from build123d import *

# Parameters (mm, degrees)
SKETCH1_R                = 13.8176
SKETCH1_R_2              = 12.7
BOSS_EXTRUDE1_DEPTH      = 16.5
SKETCH2_R                = 13.8176
BOSS_EXTRUDE2_DEPTH      = 4.318
CUT_EXTRUDE1_DEPTH       = 4.318
CIRPATTERN1_COUNT        = 6
CHAMFER1_SIZE            = 1.524
SKETCH4_R                = 4.5
BOSS_EXTRUDE3_DEPTH      = 1.5
SKETCH5_R                = 1.5875
BOSS_EXTRUDE4_DEPTH      = 0.5
BOSS_EXTRUDE4_DEPTH_BACK = 26


with BuildPart() as part:
    # Sketch1 → Boss-Extrude1 (new body)
    with BuildSketch(Plane(origin=(0, 0, 0), x_dir=(1, 0, 0), z_dir=(0, 1, 0))):
        with Locations(Location((0, 0, 0), (0, 0, 270))):  # turned: the seam where the file's is
            Circle(SKETCH1_R)
        with Locations(Location((0, 0, 0), (0, 0, 270))):  # turned: the seam where the file's is
            Circle(SKETCH1_R_2, mode=Mode.SUBTRACT)
    extrude(amount=BOSS_EXTRUDE1_DEPTH)

    # Sketch2 → Boss-Extrude2 (add)
    with BuildSketch(Plane(origin=(0, 16.5, 0), x_dir=(-1, 0, 0), z_dir=(0, 1, 0))):
        with Locations(Location((0, 0, 0), (0, 0, 90))):  # turned: the seam where the file's is
            Circle(SKETCH2_R)
    extrude(amount=-BOSS_EXTRUDE2_DEPTH)

    # Sketch3 → Cut-Extrude1 (cut)
    with BuildSketch(Plane(origin=(0, 16.5, 0), x_dir=(-1, 0, 0), z_dir=(0, 1, 0))):
        with BuildLine():
            Line((-1.905, -13.685651054), (-1.905, -6.599113577))
            ThreePointArc((-1.905, -6.599113577), (-2.8575, -4.949335183), (-4.7625, -4.949335183))
            Line((-4.7625, -4.949335183), (-10.89962148, -8.492603921))
            ThreePointArc((-10.89962148, -8.492603921), (-6.9088, -11.966392619), (-1.905, -13.685651054))
        make_face()
        with BuildLine():
            Line((-0.508, -13.808258607), (-0.508, -8.128))
            ThreePointArc((-0.508, -8.128), (-0.359210245, -7.768789755), (0, -7.62))
            Line((0, -7.62), (0, -13.8176))
            ThreePointArc((0, -13.8176), (-0.25404294, -13.815264454), (-0.508, -13.808258607))
        make_face()
        with BuildLine():
            Line((-11.704302736, -7.344070209), (-6.785054482, -4.503940905))
            ThreePointArc((-6.785054482, -4.503940905), (-6.548364162, -4.195480075), (-6.599113577, -3.81))
            Line((-6.599113577, -3.81), (-11.966392619, -6.9088))
            ThreePointArc((-11.966392619, -6.9088), (-11.837348507, -7.127639867), (-11.704302736, -7.344070209))
        make_face()
    cut_extrude1 = extrude(amount=-CUT_EXTRUDE1_DEPTH, mode=Mode.SUBTRACT)

    # CirPattern1: Cut-Extrude1 ×6 about axis
    cirpattern1_axis = Axis((0, 0, 0), (0, 1, 0))
    for i in range(1, CIRPATTERN1_COUNT):
        add(cut_extrude1.rotate(cirpattern1_axis, i * 360 / CIRPATTERN1_COUNT), mode=Mode.SUBTRACT)

    # Chamfer1
    chamfer1_edges = [part.edges().sort_by_distance(p)[0] for p in [
        (-12.524598769, 16.5, 5.83613703),
        (-11.316542312, 16.5, 7.928552191),
        (-1.208056457, 16.5, 13.764689221),
        (1.208056457, 16.5, 13.764689221),
        (1.208056457, 16.5, -13.764689221),
        (11.316542312, 16.5, 7.928552191),
        (12.524598769, 16.5, 5.83613703),
        (12.524598769, 16.5, -5.83613703),
        (11.316542312, 16.5, -7.928552191),
        (-11.316542312, 16.5, -7.928552191),
        (-12.524598769, 16.5, -5.83613703),
        (-1.208056457, 16.5, -13.764689221),
    ]]
    chamfer(chamfer1_edges, length=CHAMFER1_SIZE)

    # Sketch4 → Boss-Extrude3 (add)
    with BuildSketch(Plane(origin=(0, 16.5, 0), x_dir=(-1, 0, 0), z_dir=(0, 1, 0))):
        with Locations(Location((0, 0, 0), (0, 0, 90))):  # turned: the seam where the file's is
            Circle(SKETCH4_R)
    extrude(amount=BOSS_EXTRUDE3_DEPTH)

    # Sketch5 → Boss-Extrude4 (add, two sides)
    with BuildSketch(Plane(origin=(0, 18, 0), x_dir=(-1, 0, 0), z_dir=(0, 1, 0))) as boss_extrude4_sk:
        with Locations(Location((0, 0, 0), (0, 0, 90))):  # turned: the seam where the file's is
            Circle(SKETCH5_R)
    extrude(amount=BOSS_EXTRUDE4_DEPTH)
    extrude(boss_extrude4_sk.sketch, amount=-BOSS_EXTRUDE4_DEPTH_BACK)


solid = part.part
Build history of the part. All positions in model axes, mm. A direction names the side the tool comes from. Give positions to 0.01 mm unless a question says otherwise; leave off trailing zeros. Order: outer loops, then holes, each group sorted by start corner. A loop starts at its lowest first (then second) coordinate and runs counter-clockwise, first axis right, second up. Notation, with made-up numbers: M 88.5,63 L 124.5,63 A7 ccw 124.5,69 Z; hole C 74,31 d9. An arc over 180 degrees is marked long. Put each result on its own line as item: value.
Item 1: Wall check: probe 1 along X at (y, z) = (2.5, 0); probe 2 along Z at (x, y) = (7.5, 12.5); probe 3 along X at (y, z) = (15.75, -6.75) (3 decimals). Give the ranges that are in metal, low to high.
Results are:
probe 1: -13.82 to -12.7, -1.59 to 1.59, 12.7 to 13.82
probe 2: -6.53 to -4.92, -3.74 to -2.13, 2.13 to 3.74, 4.92 to 6.53
probe 3: -10.675 to -7.881, -1.905 to 1.905, 7.881 to 10.675
Item 2: Which spindle directions (+Z, -Z, +X, -X, +Y, -Y) get a long thin tool onto all of the face, cutting with end or side? Do faces 1 (the face through (-2.833, 14.371, 4.963)), 2 (the face through (-0.966, 2.232, -1.26)), 3 (the face through (0.508, 14, -11)), 4 (the face through (13, 12.182, 0)), 5 (the face through (9.787, 14.371, -5.064)). Say none if no direction does.
Results are:
face 1: +Z, +Y, -Y
face 2: -Y
face 3: -Z, +Y
face 4: +X, +Y
face 5: +Y
Item 3: Pull direction X, two halves, no side cores. Call faces 6 (the face through (10.61, 15.75, 7.59)), 7 (the face through (3, 16.5, -4)), 8 (the face through (0, 12.182, -13)), 9 (the face through (-11.867, 15.749, -5.417)): +X half, -X half, draft (parallel to the pull), parting line (faces both ways), or undercut.
Results are:
face 6: +X half
face 7: draft
face 8: undercut
face 9: -X half
Item 4: Cut at D-D on y = -3.5. Write the cut outline in (x, z) (1 decimal), then the cut area to 3 significant figures.
Results are:
outline: C 0,0 d3.2
area: 7.92 mm2
Item 5: Cut at A-A on z = 0. Write the cut outline in (x, y) (1 decimal), then the cut area to 3 significant figures.
Results are:
outline: M -13.8,0 L -12.7,0 L -12.7,12.2 L -13.8,12.2 Z; M -5.7,12.2 L -1.6,12.2 L -1.6,-8 L 1.6,-8 L 1.6,12.2 L 5.7,12.2 L 5.7,16.5 L 4.5,16.5 L 4.5,18 L 1.6,18 L 1.6,18.5 L -1.6,18.5 L -1.6,18 L -4.5,18 L -4.5,16.5 L -5.7,16.5 Z; M 12.7,0 L 13.8,0 L 13.8,12.2 L 12.7,12.2 Z
area: 156 mm2
Item 6: Cut at C-C on z = 10.75. Write the cut outline in (x, y) (3 decimals), then the cut area to 3 significant figures.
Results are:
outline: M -8.681,0 L -6.762,0 L -6.762,12.182 L -8.681,12.182 Z; M -1.905,12.182 L -0.508,12.182 L -0.508,16.5 L -1.905,16.5 Z; M 0.508,12.182 L 1.905,12.182 L 1.905,16.5 L 0.508,16.5 Z; M 6.762,0 L 8.681,0 L 8.681,12.182 L 6.762,12.182 Z
area: 58.8 mm2
Item 7: Drop flat-ended pins along their axis: pin 1 Ø4.5 at (x, z) = (-5.5, 11.5) entering from +Y; pin 2 Ø5 at (x, y) = (-4.5, 10.5) entering from -Z; pin 3 Ø3.5 at (y, z) = (13.5, 10) entering from +X; pin 4 Ø1 at (x, z) = (-6, 10.5) entering from +Y. Give the stop position or say it passes through.
Results are:
pin 1: y = 12.18
pin 2: z = -13.67
pin 3: x = 11.08
pin 4: through
Item 8: Cut at B-B on y = 6. Write the cut outline in (x, z) (1 decimal), then the cut area to 3 significant figures.
Results are:
outline: C 0,0 d27.6; C 0,0 d3.2; hole C 0,0 d25.4
area: 101 mm2
